```python
from build123d import *

# Parameters (mm, degrees)
F0_W      = 254
F0_H      = 177.8
F1_DEPTH  = 254
F2_W      = 24.176218
F2_H      = 76.2
F2_W_2    = 24.083782
F3_DEPTH  = 25.4
F4_W      = 33.765226
F4_H      = 33.023134
F4_W_2    = 38.217779
F4_W_3    = 34.136269
F4_H_2    = 34.507318
F4_W_4    = 51.204408
F5_DEPTH  = 254
F6_W      = 46.953924
F6_H      = 32.328948
F7_DEPTH  = 508
F8_W      = 227.147804
F8_H      = 45.486924
F8_W_2    = 42.393267
F8_H_2    = 41.027097
F8_W_3    = 63.705511
F8_H_3    = 42.462038
F8_W_4    = 41.108959
F8_H_4    = 39.725055
F9_DEPTH  = 254
F10_W     = 208.975072
F10_H     = 37.064538
F10_W_2   = 36.99249
F10_H_2   = 35.475526
F10_W_3   = 57.111204
F10_H_3   = 35.570968
F10_W_4   = 41.535424
F10_H_4   = 34.99518
F11_DEPTH = 127


with BuildPart() as f1:
    # F0 (on Front) → F1 (new body)
    with BuildSketch(Plane.XZ):
        with Locations((-1.067655, -37.961216)):
            Rectangle(F0_W, F0_H)
    extrude(amount=F1_DEPTH)

    # F2 (on Front) → F3 (cut)
    with BuildSketch(Plane.XZ):
        with Locations((-12.088109, -92.779977)):
            Rectangle(F2_W, F2_H)
        with Locations((12.041891, -92.779977)):
            Rectangle(F2_W_2, F2_H)
    extrude(amount=F3_DEPTH, mode=Mode.SUBTRACT)

    # F4 (on Front) → F5 (cut)
    with BuildSketch(Plane.XZ):
        with Locations((-69.497861, -72.430827)):
            Rectangle(F4_W, F4_H)
        with Locations((72.983959, -72.430827)):
            Rectangle(F4_W_2, F4_H)
        with Locations((75.024715, -7.868753)):
            Rectangle(F4_W_3, F4_H_2)
        with Locations((-69.497861, -7.868753)):
            Rectangle(F4_W, F4_H_2)
        with Locations((-0.668756, -7.868753)):
            Rectangle(F4_W_4, F4_H_2)
    extrude(amount=F5_DEPTH, mode=Mode.SUBTRACT)

    # F6 (on Front) → F7 (cut)
    with BuildSketch(Plane.XZ):
        with Locations((-0.388555, -74.189298)):
            Rectangle(F6_W, F6_H)
    extrude(amount=F7_DEPTH, mode=Mode.SUBTRACT)

    # F8 (on Right) → F9 (cut)
    with BuildSketch(Plane.YZ):
        with Locations((-123.347826, -77.906983)):
            Rectangle(F8_W, F8_H)
        with Locations((-210.81461, -11.680585)):
            Rectangle(F8_W_2, F8_H_2)
        with Locations((-129.083659, -11.576193)):
            Rectangle(F8_W_3, F8_H_3)
        with Locations((-52.509461, -9.497304)):
            Rectangle(F8_W_4, F8_H_4)
    extrude(amount=-F9_DEPTH, mode=Mode.SUBTRACT)

    # F10 (on Right) → F11 (cut)
    with BuildSketch(Plane.YZ):
        with Locations((-115.409213, -79.144068)):
            Rectangle(F10_W, F10_H)
        with Locations((-185.175732, -17.737763)):
            Rectangle(F10_W_2, F10_H_2)
        with Locations((-111.515269, -17.785484)):
            Rectangle(F10_W_3, F10_H_3)
        with Locations((-42.073241, -17.49759)):
            Rectangle(F10_W_4, F10_H_4)
    extrude(amount=F11_DEPTH, mode=Mode.SUBTRACT)


solid = f1.part
```
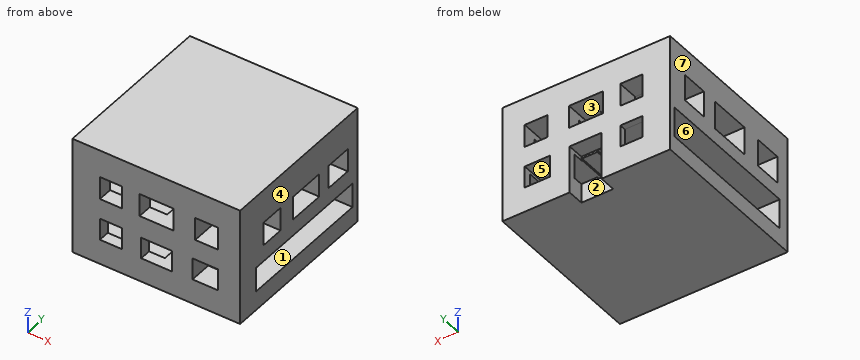
Can you work these out from the model? Positions are in its coordinate system, mm. Face numbers are marked on the shaded views. A direction names the side the tool comes from. Give positions to 0.01 mm unless a question says otherwise; leave off trailing zeros. Write each loop counter-clockwise with the first axis right and the second up, starting at its lowest first coordinate (ties: lowest second). Pieces come first, ordered by that corner, then holes. Notation, with made-up numbers: (16.5, 8) -> (63.5, 8) arc R16 cw to (63.5, 24) -> close; hole circle Ø7 at (-9, 29). An arc over 180 degrees is marked (long way). One line per item, written item: value.
Q1. For P1, Ø12, axis at y = -84.5, z = -11, coming from the +X side, with a flat end and sliding along its axis, tell me the tip position at first contact or that it passes through.
Results found:
P1: stops at x = 125.93
Q2. Please list where these lines run through material, in increasing order: line 1 (Z direction, x = 65, y = -106); line 2 (Z direction, x = -104, y = -209.5); line 3 (Y direction, x = -49.5, z = -16). Write a range as [from, to].
Results found:
line 1: z = [-126.86, -97.68], [-55.92, -35.57], [9.38, 50.94]
line 2: z = [-126.86, -100.65], [-55.16, -32.19], [8.83, 50.94]
line 3: y = [-254, -232.01], [-189.62, -160.94], [-97.23, -73.06], [-31.95, 0]
Q3. Which directions (+Z, -Z, +X, -X, +Y, -Y) give clear straight access to the entire face, cutting with the end or side of a thin tool? Please do the marked faces 1, 2 and 3.
Results found:
face 1: +X, -X
face 2: -Z, +Y
face 3: +Y, -Y
Q4. We'd pull the mould along X, two halves only. Please class the marked faces 4, 5, 6 and 7: +X half, -X half, draft (parallel to the pull), parting line (faces both ways), or undercut.
Results found:
face 4: +X half
face 5: undercut
face 6: draft
face 7: -X half
Q5. Imagine slicing it at C-C on x = 79. Please give me the cut outline in (y, z).
Results found:
outline: (-254, -126.86) -> (0, -126.86) -> (0, -88.94) -> (-10.92, -88.94) -> (-10.92, -97.68) -> (-219.9, -97.68) -> (-219.9, -88.94) -> (-254, -88.94) -> close; (-254, -55.92) -> (0, -55.92) -> (0, -25.12) -> (-21.31, -25.12) -> (-21.31, -35) -> (-62.84, -35) -> (-62.84, -25.12) -> (-82.96, -25.12) -> (-82.96, -35.57) -> (-140.07, -35.57) -> (-140.07, -25.12) -> (-166.68, -25.12) -> (-166.68, -35.48) -> (-203.67, -35.48) -> (-203.67, -25.12) -> (-254, -25.12) -> close; (-254, 9.38) -> (0, 9.38) -> (0, 50.94) -> (-254, 50.94) -> close
Q6. Imagine slicing it at A-A on y = -67. Give the number of separate pieces and of enclosed holes in the cut face, and give its area (3 significant figures).
Results found:
separate pieces: 2
enclosed holes: 1
area: 27,300 mm^2
